Job drawing, mm, ordinate dimensions from the low corner. One solid piece. Round coordinates to 2 decimals unless told otherwise and drop trailing zeros. Write each loop counter-clockwise with the first axis right and the second up, starting at its lowest first coordinate (ties: lowest second). Pieces come first, ordered by that corner, then holes.
1) Saw through at A-A on z = 3.8. Write the cut outline in (x, y), and give its area (3 significant figures).
2) Saw through at D-D on x = 4.5. Write the cut outline in (y, z).
3) Drill centre lines: L1, parallel to Y at x = 41, z = 4.1; L2, parallel to X at y = 40.5, z = 5.3; L3, parallel to Y at x = 20.5, z = 5.4. Where is each one in solid material? Low to high.
4) Saw through at C-C on y = 18.5. Write the cut outline in (x, z).
5) Flat gauge pins, fed straight in: pin 1 (0.5 mm diameter, centred on y = 40, z = 5.5, fed in from -X); pin 2 (1 mm diameter, centred on y = 68, z = 2.5, fed in from -X); pin 3 (5 mm diameter, centred on x = 40.92, y = 67.29, fed in from +Z); pin 4 (0.5 mm diameter, centred on x = 27.5, z = 5.5, fed in from -Y). Where does each tip first touch, or does it go through?
6) Saw through at B-B on x = 19. Write the cut outline in (y, z), and give its area (3 significant figures).
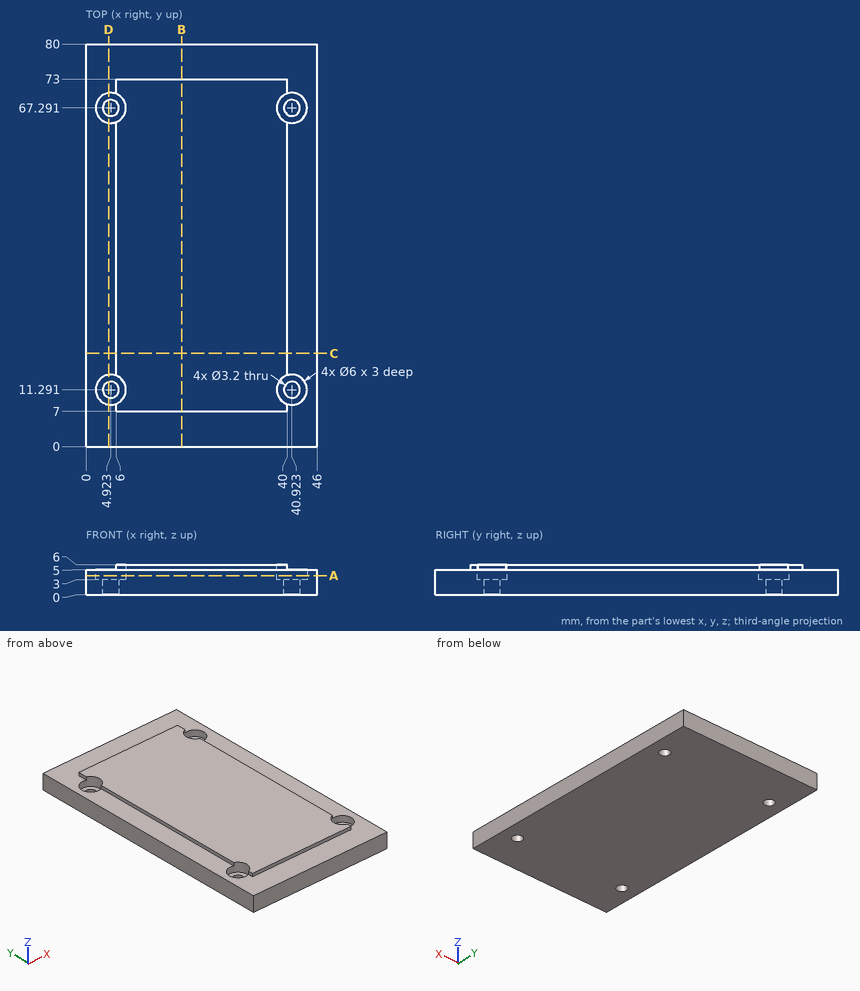
Completed:
1. outline: (0, 0) - (46, 0) - (46, 80) - (0, 80) - close; hole circle Ø6 at (4.92, 11.29); hole circle Ø6 at (4.92, 67.29); hole circle Ø6 at (40.92, 11.29); hole circle Ø6 at (40.92, 67.29)
1. area: 3,570 mm2
2. outline: (0, 0) - (9.75, 0) - (9.75, 3) - (8.32, 3) - (8.32, 5) - (0, 5) - close; (12.83, 0) - (65.75, 0) - (65.75, 3) - (64.32, 3) - (64.32, 5) - (14.26, 5) - (14.26, 3) - (12.83, 3) - close; (68.83, 0) - (80, 0) - (80, 5) - (70.26, 5) - (70.26, 3) - (68.83, 3) - close
3. L1: y = 0 to 8.29, 14.29 to 64.29, 70.29 to 80
3. L2: x = 6 to 40
3. L3: y = 7 to 73
4. outline: (0, 0) - (46, 0) - (46, 5) - (40, 5) - (40, 6) - (6, 6) - (6, 5) - (0, 5) - close
5. pin 1: stops at x = 6
5. pin 2: stops at x = 0
5. pin 3: stops at z = 3
5. pin 4: stops at y = 7
6. outline: (0, 0) - (80, 0) - (80, 5) - (73, 5) - (73, 6) - (7, 6) - (7, 5) - (0, 5) - close
6. area: 466 mm2
